```python
from build123d import *

# Parameters (mm, degrees)
SKETCH_W     = 120
SKETCH_H     = 120
SKETCH_R     = 2.25
SKETCH_R_2   = 24
PAD_DEPTH    = 5
FILLET_R     = 4
CHAMFER_SIZE = 4


with BuildPart() as part:
    # Sketch → Pad (new body)
    with BuildSketch(Plane.XY):
        Rectangle(SKETCH_W, SKETCH_H)
        with Locations((-55, 55)):
            Circle(SKETCH_R, mode=Mode.SUBTRACT)
        with Locations((55, 55)):
            Circle(SKETCH_R, mode=Mode.SUBTRACT)
        with Locations((55, -55)):
            Circle(SKETCH_R, mode=Mode.SUBTRACT)
        with Locations((-55, -55)):
            Circle(SKETCH_R, mode=Mode.SUBTRACT)
        Circle(SKETCH_R_2, mode=Mode.SUBTRACT)
    extrude(amount=PAD_DEPTH)

    # Fillet
    fillet_edges = [part.edges().sort_by_distance(p)[0] for p in [
        (-24, 0, 0),
    ]]
    fillet(fillet_edges, radius=FILLET_R)

    # Chamfer
    chamfer_edges = [part.edges().sort_by_distance(p)[0] for p in [
        (-60, -60, 2.5),
        (60, -60, 2.5),
        (60, 60, 2.5),
        (-60, 60, 2.5),
    ]]
    chamfer(chamfer_edges, length=CHAMFER_SIZE)


solid = part.part
```
Design review of the part built by this model. Coordinates are the model's own, in mm. Coordinates: 2 decimals unless noted, no trailing zeros. Order: outer loops, then holes, each group sorted by start corner. A loop starts at its lowest first (then second) coordinate and runs counter-clockwise, first axis right, second up. Notation, with made-up numbers: M 5,26.5 L 56,26.5 A30 ccw 56,55.5 Z; hole C 41.25,-5.75 d9. An arc over 180 degrees is marked long. Answer as a JSON object with one key per item and string values. Group by question number.
1) Add section A-A, the plane y = 0. Write out the cut boundary in (x, z), then the cut area to 3 significant figures.
2) Wall thickness on L1, parallel to Y at x = -55, z = 2; L2, parallel to Y at x = 0, z = 4.4; L3, parallel to X at y = 54, z = 3: over which ranges is each line inside the solid? List them lowest first.
3) Mouldability with a two-part tool opening along Y and no side actions: class faces 1 (the cylindrical face through (-57.248, -54.901, 2.465)), 2 (the flat face through (-1, 60, 2)), 3 (the flat face through (-58, -58, 2)) as pulls with the +Y half, pulls with the -Y half, needs draft (parallel to the pull), parting line crosses it, or undercut.
4) For pin 1 (4 mm diameter, centred on x = 12, y = -42.5, fed in from -Z); pin 2 (2.5 mm diameter, centred on x = 55, y = -55, fed in from +Z), all flat-tipped, find the tip position at first contact; note any pin that passes through.
5) Add section B-B, the plane z = 2.7. Write out the cut boundary in (x, y).
Computed values:
{
 "1": {"outline": "M -60,0 L -28,0 A4 ccw -24,4 L -24,5 L -60,5 Z; M 24,4 A4 ccw 28,0 L 60,0 L 60,5 L 24,5 Z", "area": "353 mm^2"},
 "2": {"L1": "y = -60 to -57.25, -52.75 to 52.75, 57.25 to 60", "L2": "y = -60 to -24, 24 to 60", "L3": "x = -60 to -57.02, -52.98 to 52.98, 57.02 to 60"},
 "3": {"face 1": "undercut", "face 2": "pulls with the +Y half", "face 3": "pulls with the -Y half"},
 "4": {"pin 1": "stops at z = 0", "pin 2": "passes through"},
 "5": {"outline": "M -60,-56 L -56,-60 L 56,-60 L 60,-56 L 60,56 L 56,60 L -56,60 L -60,56 Z; hole C -55,-55 d4.5; hole C -55,55 d4.5; hole C 0,0 d48.43; hole C 55,-55 d4.5; hole C 55,55 d4.5"}
}
